```python
from build123d import *

# Parameters (mm, degrees)
COVER_FRAME_W                 = 150
COVER_FRAME_H                 = 87
COVER_THICKNESS_DEPTH         = 3
COVER_ITEMS_MOUTING_HOLES_R   = 2.5
COVER_ITEMS_MOUTING_HOLES_R_2 = 1
COVER_ITEMS_MOUTING_HOLES_R_3 = 1.75
COVER_ITEMS_HOLES_DEPTH       = 5
COVER_SCREW_HOLES_R           = 1
COVER_SCREW_DEPTH             = 9
COVER_EDGES_R                 = 3
SKETCH10_W                    = 37
SKETCH10_H                    = 37
LOAD_OUTLET_DEPTH             = 9
SKETCH11_R                    = 2.8
INDICATOR_LEDS_DEPTH          = 4
SKETCH12_W                    = 72
SKETCH12_H                    = 25
LCD_DEPTH                     = 4
SKETCH13_R                    = 2.5
COVER_SCREW_COUNTERSUNK_DEPTH = 1.5


with BuildPart() as part:
    # Cover_frame → cover_thickness (new body)
    with BuildSketch(Plane(origin=(0, 0, 0), x_dir=(1, 0, 0), z_dir=(0, 1, 0))):
        with Locations((75, 43.5)):
            Rectangle(COVER_FRAME_W, COVER_FRAME_H)
    extrude(amount=COVER_THICKNESS_DEPTH)

    # cover_items_mouting_holes → cover_items_holes (add)
    with BuildSketch(Plane.XZ):
        with Locations((15.5, -76.5)):
            Circle(COVER_ITEMS_MOUTING_HOLES_R)
        with Locations((15.5, -76.5)):
            Circle(COVER_ITEMS_MOUTING_HOLES_R_2, mode=Mode.SUBTRACT)
        with Locations((15.5, -45.5)):
            Circle(COVER_ITEMS_MOUTING_HOLES_R_3)
        with Locations((15.5, -45.5)):
            Circle(COVER_ITEMS_MOUTING_HOLES_R_2, mode=Mode.SUBTRACT)
        with Locations((90.5, -76.5)):
            Circle(COVER_ITEMS_MOUTING_HOLES_R)
        with Locations((90.5, -76.5)):
            Circle(COVER_ITEMS_MOUTING_HOLES_R_2, mode=Mode.SUBTRACT)
        with Locations((90.5, -45.5)):
            Circle(COVER_ITEMS_MOUTING_HOLES_R)
        with Locations((90.5, -45.5)):
            Circle(COVER_ITEMS_MOUTING_HOLES_R_2, mode=Mode.SUBTRACT)
        with Locations((15.5, -35.5)):
            Circle(COVER_ITEMS_MOUTING_HOLES_R)
        with Locations((15.5, -35.5)):
            Circle(COVER_ITEMS_MOUTING_HOLES_R_2, mode=Mode.SUBTRACT)
        with Locations((15.5, -10.5)):
            Circle(COVER_ITEMS_MOUTING_HOLES_R)
        with Locations((15.5, -10.5)):
            Circle(COVER_ITEMS_MOUTING_HOLES_R_2, mode=Mode.SUBTRACT)
        with Locations((84.5, -35.5)):
            Circle(COVER_ITEMS_MOUTING_HOLES_R)
        with Locations((84.5, -35.5)):
            Circle(COVER_ITEMS_MOUTING_HOLES_R_2, mode=Mode.SUBTRACT)
        with Locations((84.5, -10.5)):
            Circle(COVER_ITEMS_MOUTING_HOLES_R)
        with Locations((84.5, -10.5)):
            Circle(COVER_ITEMS_MOUTING_HOLES_R_2, mode=Mode.SUBTRACT)
    extrude(amount=COVER_ITEMS_HOLES_DEPTH)

    # Cover_screw_holes → cover_screw (cut, through all)
    with BuildSketch(Plane(origin=(0, 3, 0), x_dir=(1, 0, 0), z_dir=(0, 1, 0))):
        with Locations((5.5, 81.5)):
            Circle(COVER_SCREW_HOLES_R)
        with Locations((5.5, 5.5)):
            Circle(COVER_SCREW_HOLES_R)
    cover_screw = extrude(amount=-COVER_SCREW_DEPTH, mode=Mode.SUBTRACT)

    # Mirror2: cover_screw across plane
    add(cover_screw.mirror(Plane.ZY.offset(-75)), mode=Mode.SUBTRACT)

    # cover_edges
    cover_edges_edges = [part.edges().sort_by_distance(p)[0] for p in [
        (0, 1.5, -87),
        (150, 1.5, -87),
        (150, 1.5, 0),
        (0, 1.5, 0),
    ]]
    fillet(cover_edges_edges, radius=COVER_EDGES_R)

    # Sketch10 → Load_outlet (cut, through all)
    with BuildSketch(Plane(origin=(0, 3, 0), x_dir=(1, 0, 0), z_dir=(0, 1, 0))):
        with Locations((120.5, 60.5)):
            Rectangle(SKETCH10_W, SKETCH10_H)
    extrude(amount=-LOAD_OUTLET_DEPTH, mode=Mode.SUBTRACT)

    # Sketch11 → Indicator_leds (cut, through all)
    with BuildSketch(Plane.XZ):
        with Locations((67.25, -23)):
            Circle(SKETCH11_R)
        with Locations((32.75, -23)):
            Circle(SKETCH11_R)
    extrude(amount=-INDICATOR_LEDS_DEPTH, mode=Mode.SUBTRACT)

    # Sketch12 → LCD (cut, through all)
    with BuildSketch(Plane.XZ):
        with Locations((52.5, -60)):
            Rectangle(SKETCH12_W, SKETCH12_H)
    extrude(amount=-LCD_DEPTH, mode=Mode.SUBTRACT)

    # Sketch13 → cover_screw_countersunk (cut)
    with BuildSketch(Plane(origin=(0, 3, 0), x_dir=(1, 0, 0), z_dir=(0, 1, 0))):
        with Locations((5.5, 81.5)):
            Circle(SKETCH13_R)
        with Locations((5.5, 5.5)):
            Circle(SKETCH13_R)
    cover_screw_countersunk = extrude(amount=-COVER_SCREW_COUNTERSUNK_DEPTH, mode=Mode.SUBTRACT)

    # Mirror3: cover_screw_countersunk across plane
    add(cover_screw_countersunk.mirror(Plane.ZY.offset(-75)), mode=Mode.SUBTRACT)


solid = part.part
```
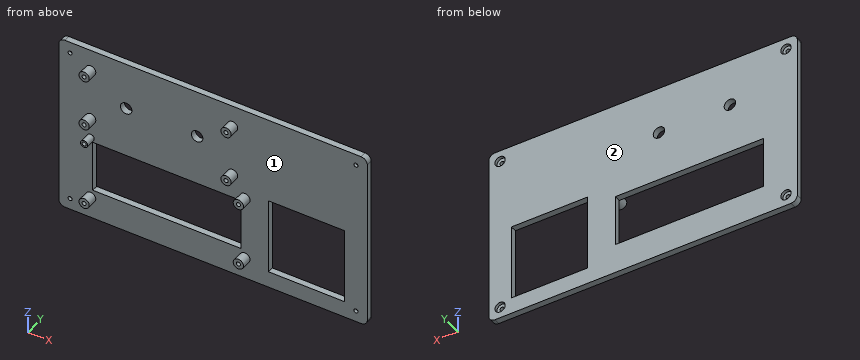
Check sheet for the modelled part. Datum: model origin and axes. Units: mm. Face numbers are marked on the shaded views. Give positions to 0.01 mm unless a question says otherwise; leave off trailing zeros. Write each loop counter-clockwise with the first axis right and the second up, starting at its lowest first coordinate (ties: lowest second). Pieces come first, ordered by that corner, then holes.
Item 1: Cross-section at C-C (z = -60.5). Enter the section's corners in (x, y), and give its area (3 significant figures).
Item 2: Cross-section at A-A (y = -1.75). Count the separate pieces of the cut face and the enclosed holes in it, and give its area (3 significant figures).
Item 3: Scan lines: L1, parallel to Z at x = 144.5, y = 2.45; L2, parallel to Z at x = 90.5, y = -1.8; L3, parallel to X at y = 2.4, z = -81.5. Record each from-to range of solid material in increasing order.
Item 4: Cross-section at D-D (x = 137). Enter the section's corners in (y, z).
Item 5: Draft check along X on the marked faces 1 and 2. Enter one of: released by +X, released by -X, zero draft, split by the parting line, or undercut.
Item 6: Cross-section at B-B (x = 32.75). Enter the section's corners in (y, z).
Item 7: Gauge pin test, flat ends, axial feed: pin 1 (4 mm diameter, centred on x = 65, z = -77, fed in from -Y); pin 2 (2.5 mm diameter, centred on x = 5.5, z = -5.5, fed in from +Y); pin 3 (4 mm diameter, centred on x = 4.5, z = -5, fed in from +Y); pin 4 (1.2 mm diameter, centred on x = 144.5, z = -81.5, fed in from +Y). Record the tip position at first contact, or that the pin passes through.
Report:
1. outline: (0, 0) - (16.5, 0) - (16.5, 3) - (0, 3) - close; (88.5, 0) - (102, 0) - (102, 3) - (88.5, 3) - close; (139, 0) - (150, 0) - (150, 3) - (139, 3) - close
1. area: 123 mm2
2. separate pieces: 8
2. enclosed holes: 8
2. area: 122 mm2
3. L1: z = -87 to -84, -79 to -8, -3 to 0
3. L2: z = -79 to -77.5, -75.5 to -74, -48 to -46.5, -44.5 to -43
3. L3: x = 0 to 3, 8 to 142, 147 to 150
4. outline: (0, -87) - (3, -87) - (3, -79) - (0, -79) - close; (0, -42) - (3, -42) - (3, 0) - (0, 0) - close
5. face 1: undercut
5. face 2: zero draft
6. outline: (0, -87) - (3, -87) - (3, -72.5) - (0, -72.5) - close; (0, -47.5) - (3, -47.5) - (3, -25.8) - (0, -25.8) - close; (0, -20.2) - (3, -20.2) - (3, 0) - (0, 0) - close
7. pin 1: stops at y = 0
7. pin 2: stops at y = 1.5
7. pin 3: stops at y = 3
7. pin 4: passes through
